The listing builds one solid part. Answer for the finished solid, in the listing's coordinates (mm). Round coordinates to 2 decimals unless told otherwise and drop trailing zeros. Order: outer loops, then holes, each group sorted by start corner. A loop starts at its lowest first (then second) coordinate and runs counter-clockwise, first axis right, second up. Notation, with made-up numbers: (75.25, 88.25) - (94.25, 88.25) arc R4 cw to (94.25, 94.25) - close; hole circle Ø9 at (-40, 39.5). An arc over 180 degrees is marked (long way). Write item = value, one per line.
Autodesk Fusion 360 part; units mm, degrees
sketch "Sketch1" plane through (0, 0, 0) normal (0, 0, 1) x (1, 0, 0)
  line L0 (30, 30) -> (-30, 30)
  line L1 (-30, 30) -> (-30, -30)
  line L2 (-30, -30) -> (30, -30)
  line L3 (30, -30) -> (30, 30)
  line L4 (30, 30) -> (-30, -30) construction
  line L5 (-30, 30) -> (30, -30) construction
  line L6 (-30, -30) -> (-15, -30) construction
  line L7 (-15, -30) -> (-15, -15) construction
  line L8 (-15, -15) -> (-30, -15) construction
  line L9 (-30, -15) -> (-30, -30) construction
  line L10 (-11, -3) -> (-19, -3)
  line L11 (-19, -3) -> (-19, -27)
  line L12 (-19, -27) -> (-11, -27)
  line L13 (-11, -27) -> (-11, -3)
  line L14 (-11, -3) -> (-19, -27) construction
  line L15 (-19, -3) -> (-11, -27) construction
  line L16 (-11, -7) -> (-19, -7)
  line L17 (-19, -7) -> (-19, -23)
  line L18 (-19, -23) -> (-11, -23)
  line L19 (-11, -23) -> (-11, -7)
  line L20 (-11, -7) -> (-19, -23) construction
  line L21 (-19, -7) -> (-11, -23) construction
  point P0 (-15, -15)
  point P1 (-15, -15)
  point P2 (-15, -15)
  dimension "d1" = 60
  dimension "d2" = 60
  dimension "d25" = 15
  dimension "d26" = 15
  dimension "d38" = 8
  dimension "d39" = 24
  dimension "d40" = 8
  dimension "d41" = 16
extrude "Extrude1" add sketch "Sketch1" against normal blind 4 contours L0 L1 L2 L3 | L10 L11 L13 L16 | L11 L13 L16 L17 L18 L19 | L11 L12 L13 L18 in component "body"
hole "Hole2" at (-15, -15, 0) direction (0, 0, -1) diameter 6 depth 4 tip angle 118 counterbore diameter 11.5 counterbore depth 1 in component "body"
extrude "Extrude2" add sketch "Sketch1" against normal blind 2 from surface at -4 contours L10 L11 L13 L16 | L11 L12 L13 L18 in component "body"
chamfer "Chamfer4" distance 0.5 angle 45 2 faces at (-16.3333, -25.6667, -6) (-16.3333, -4.3333, -6) in component "body"
chamfer "Chamfer4" distance 0.6 angle 45 1 edges at (-20.3609, -12.9207, 0) in component "body"
pattern_linear "R-Pattern2" count 2 spacing 30 along (0, 1, 0) count 2 spacing 30 along (1, 0, 0) of "Hole2", "Extrude2", "Chamfer4" in component "body"
fillet "Fillet1" radius 2 4 edges at (-30, -30, -2) (30, -30, -2) (30, 30, -2) (-30, 30, -2) in component "body"
chamfer "Chamfer1" distance 1 distance2 1 8 edges at (0, -30, 0) (29.4142, -29.4142, 0) (30, 0, 0) (29.4142, 29.4142, 0) (0, 30, 0) (-29.4142, 29.4142, 0) (-30, 0, 0) (-29.4142, -29.4142, 0) measured on face at (-3.5603, 3.4484, 0) measured on face at (28.0952, -29.9977, -1.3333) measured on face at (-3.5603, 3.4484, 0) measured on face at (28.0952, 29.9977, -1.3333) measured on face at (-3.5603, 3.4484, 0) measured on face at (-29.9977, 28.0952, -1.3333) measured on face at (-3.5603, 3.4484, 0) measured on face at (-29.9977, -28.0952, -1.3333) in component "body"
component "body" placed x (1, 0, 0) y (0, 1, 0) z (0, 0, 1) at (0, 0, 0)
equation "d2 = unitY * size"
equation "size = 30 mm"
equation "d23 = size"
equation "d25 = size / 2"
equation "d26 = size / 2"
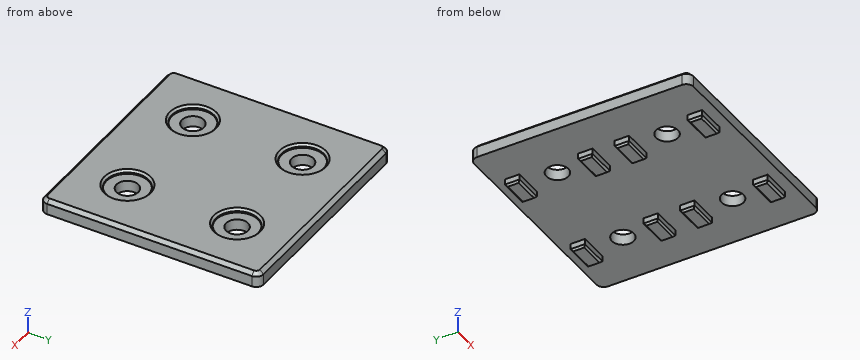
Q1. Section A-A on y = -15 is taken. Determine the outline of the cut face in (x, z).
Model answer:
outline = (-30, -4) - (-18, -4) - (-18, -1) - (-20.75, -1) - (-20.75, -0.6) - (-21.35, 0) - (-29, 0) - (-30, -1) - close; (-12, -4) - (12, -4) - (12, -1) - (9.25, -1) - (9.25, -0.6) - (8.65, 0) - (-8.65, 0) - (-9.25, -0.6) - (-9.25, -1) - (-12, -1) - close; (18, -4) - (30, -4) - (30, -1) - (29, 0) - (21.35, 0) - (20.75, -0.6) - (20.75, -1) - (18, -1) - close
Q2. Section C-C on x = -15 is taken. Count the separate pieces of the cut face and the enclosed holes in it, then the cut area to 3 significant figures.
Model answer:
separate_pieces = 3
enclosed_holes = 0
area = 210 mm^2
Q3. Section D-D on x = 3.5 is taken. Determine the outline of the cut face in (y, z).
Model answer:
outline = (-30, -4) - (30, -4) - (30, -1) - (29, 0) - (-29, 0) - (-30, -1) - close
Q4. Section B-B on z = -2.5 is taken. Determine the outline of the cut face in (x, y).
Model answer:
outline = (-30, -28) arc R2 ccw to (-28, -30) - (28, -30) arc R2 ccw to (30, -28) - (30, 28) arc R2 ccw to (28, 30) - (-28, 30) arc R2 ccw to (-30, 28) - close; hole circle Ø6 at (-15, -15); hole circle Ø6 at (-15, 15); hole circle Ø6 at (15, -15); hole circle Ø6 at (15, 15)
Q5. Find the intervals of material crossed by line 1 (X direction, y = 25, z = -5.5); line 2 (X direction, y = -15, z = -2.75); line 3 (Y direction, x = -15, z = -0.85), in increasing order. Write a range as from..to.
Model answer:
line_1 = -19..-11, 11..19
line_2 = -30..-18, -12..12, 18..30
line_3 = -29.85..-20.75, -9.25..9.25, 20.75..29.85
Q6. Flat-ended cylindrical pins translate along their axes: P1, Ø0.8, axis at y = -5, z = -5, coming from the -X side; P2, Ø3, axis at y = -3.5, z = -4.5, coming from the -X side; P3, Ø1.6, axis at y = -5.5, z = -5, coming from the +X side; P4, Ø1.5, axis at x = -1, y = -9.5, coming from the -Z side. Find the tip coordinate at first contact, or state that the pin passes through.
Model answer:
P1 = -19
P2 = -30
P3 = 19
P4 = -4
